Check sheet for the modelled part. Datum: model origin and axes. Units: mm. A direction names the side the tool comes from. Give positions to 0.01 mm unless a question says otherwise; leave off trailing zeros. Write each loop counter-clockwise with the first axis right and the second up, starting at its lowest first coordinate (ties: lowest second). Pieces come first, ordered by that corner, then holes. Notation, with made-up numbers: M 61.5,81 L 104.5,81 A31 ccw 104.5,109 Z; hole C 37.25,-18 d1. An arc over 180 degrees is marked long. Write item = value, one per line. Start each with the question number.
1) Mould release check, pull along X, two halves, no side actions. Record for faces 4 (the flat face through (-15, 0, 0)), 5 (the cylindrical face through (-14.6, 0.07, 1.57)): released by +X, released by -X, zero draft, split by the parting line, or undercut.
2) Cross-section at B-B, the plane z = 1.2. Give the number of separate pieces and of enclosed holes in the cut face, plus the area to 3 significant figures.
3) Scan lines: line 1 along Y through (x, z) = (-23, 1.5); line 2 along X through (y, z) = (0.75, 1.4); line 3 along X through (y, z) = (-1, 0.4). Record each from-to range of solid material in increasing order. Write a range as [from, to].
4) Go/stop test with flat-tipped pins: pin 1 (1.5 mm diameter, centred on x = -16, y = -6, fed in from -Z); pin 2 (1 mm diameter, centred on x = -13.5, z = 1, fed in from +Y); pin 3 (1 mm diameter, centred on x = -23, z = 1.5, fed in from -Y); pin 4 (1 mm diameter, centred on x = -7, y = -1, fed in from -Z). Record where each tip stops, or that it passes through.
5) Cross-section at C-C, the plane y = 5.5. Record the cut outline in (x, z) (3 decimals), plus the area to 3 significant figures.
6) Cross-section at D-D, the plane x = -30.5. Record the cut outline in (y, z) (3 decimals), plus the area to 4 significant figures.
7) Cross-section at A-A, the plane x = -13. Record the cut outline in (y, z) (3 decimals).
8) Access from +Z, -Z, +X, -X, +Y, -Y to the whole of each face (thin tool, end or side, straight path). Record for faces 1 (the flat face through (-19, -5, 2)), 2 (the flat face through (-15, 0, 3.175)), 3 (the flat face through (-19, 5, 2)).
```python
from build123d import *

# Parameters (mm, degrees)
F0_R     = 1.6
F1_DEPTH = 3.175


with BuildPart() as f1:
    # F0 (on Top) → F1 (new body)
    with BuildSketch(Plane.XY):
        with BuildLine():
            ThreePointArc((7.5, 0), (2.6761656733, 7.0062926922), (-5.5901699437, 5))
            Line((-5.5901699437, 5), (-32.6, 5))
            ThreePointArc((-32.6, 5), (-36.1355339059, 3.5355339059), (-37.6, 0))
            ThreePointArc((-37.6, 0), (-36.1355339059, -3.5355339059), (-32.6, -5))
            Line((-32.6, -5), (-5.5901699437, -5))
            ThreePointArc((-5.5901699437, -5), (2.6761656733, -7.0062926922), (7.5, 0))
        make_face()
        with Locations((-33, 0)):
            Circle(F0_R, mode=Mode.SUBTRACT)
        with Locations((-23, 0)):
            Circle(F0_R, mode=Mode.SUBTRACT)
        with Locations((-13, 0)):
            Circle(F0_R, mode=Mode.SUBTRACT)
        Polygon((-2.3131272616, 1.150841372), (-2.4811892868, 1.651717782), (-1.9542535042, 1.6899369317), (-1.992472654, 2.2168727143), (-1.4725868119, 2.1228475389), (-1.3785616365, 2.6427333809), (-0.8983920744, 2.4223718279), (-0.6780305213, 2.90254139), (-0.2677480588, 2.5696895861), (0.0651037451, 2.9799720486), (0.379719552, 2.555544297), (0.8041473037, 2.8701601039), (1.0033279869, 2.380824761), (1.4926633298, 2.5800054442), (1.5638936344, 2.0565092492), (2.0873898293, 2.1277395538), (2.0261940932, 1.6029756981), (2.5509579489, 1.5417799619), (2.3611813253, 1.0487212884), (2.8542399989, 0.8589446648), (2.547806851, 0.4285718633), (2.9781796525, 0.1221387154), (2.574344302, -0.2185063082), (2.9149893256, -0.6223416587), (2.4391262327, -0.8518549247), (2.6686394987, -1.3277180175), (2.1506488918, -1.4316783634), (2.2546092377, -1.9496689703), (1.7270383715, -1.9215441851), (1.6989135863, -2.4491150513), (1.1949116786, -2.2906723188), (1.0364689461, -2.7946742265), (0.5877042905, -2.5158690862), (0.3088991502, -2.9646337418), (-0.0564307197, -2.5829845462), (-0.4380799154, -2.9483144161), (-0.6970199802, -2.4878015876), (-1.1575328087, -2.7467416524), (-1.2938129119, -2.2363009057), (-1.8042536586, -2.3725810089), (-1.80931082, -1.8442852134), (-2.3376066155, -1.8493423749), (-2.2111230752, -1.3363862984), (-2.7240791517, -1.209902758), (-2.4740023355, -0.7445173173), (-2.9393877762, -0.4944405012), (-2.5814309304, -0.105867575), (-2.9700038565, 0.2520892708), (-2.5266587261, 0.5394342163), (-2.8140036716, 0.9827793468), align=None, mode=Mode.SUBTRACT)
    extrude(amount=F1_DEPTH)


solid = f1.part
```
Reply:
q1.face_4 = zero draft
q1.face_5 = undercut
q2.separate_pieces = 1
q2.enclosed_holes = 4
q2.area = 425 mm2
q3.line_1 = [-5, -1.6], [1.6, 5]
q3.line_2 = [-37.54, -34.41], [-31.59, -24.41], [-21.59, -14.41], [-11.59, -2.66], [2.78, 7.46]
q3.line_3 = [-37.5, -34.25], [-31.75, -24.25], [-21.75, -14.25], [-11.75, -2.61], [2.51, 7.43]
q4.pin_1 = through
q4.pin_2 = 5
q4.pin_3 = -5
q4.pin_4 = 0
q5.outline = M -5.099,0 L 5.099,0 L 5.099,3.175 L -5.099,3.175 Z
q5.area = 32.4 mm2
q6.outline = M -5,0 L 5,0 L 5,3.175 L -5,3.175 Z
q6.area = 31.75 mm2
q7.outline = M -5,0 L -1.6,0 L -1.6,3.175 L -5,3.175 Z; M 1.6,0 L 5,0 L 5,3.175 L 1.6,3.175 Z
q8.face_1 = +Z, -Z, -X, -Y
q8.face_2 = +Z, +X, -X, +Y, -Y
q8.face_3 = +Z, -Z, -X, +Y
